```python
from build123d import *

# Parameters (mm, degrees)
BOSS_EXTRUDE1_DEPTH        = 40.48125
SKETCH3_R                  = 6.35
BOSS_EXTRUDE2_DEPTH        = 7.9375
F_10_32_TAPPED_HOLE1_D     = 4.0386
F_10_32_TAPPED_HOLE1_DEPTH = 12.02944
F_10_32_TAPPED_HOLE1_TIP   = 1.213317848
SKETCH2_R                  = 2.0193
CUT_EXTRUDE1_DEPTH         = 90.388013306


with BuildPart() as part:
    # Sketch1 → Boss-Extrude1 (new, symmetric)
    with BuildSketch(Plane(origin=(0, 0, 0), x_dir=(1, 0, 0), z_dir=(0, 1, 0))):
        with BuildLine():
            ThreePointArc((0.990636919, 6.760403927), (0, 6.8326), (-0.990636919, 6.760403927))
            Line((-0.990636919, 6.760403927), (-5.359363081, 4.238118701))
            ThreePointArc((-5.359363081, 4.238118701), (-5.917205174, 3.4163), (-6.35, 2.522285226))
            Line((-6.35, 2.522285226), (-6.35, -2.522285226))
            ThreePointArc((-6.35, -2.522285226), (-5.917205174, -3.4163), (-5.359363081, -4.238118701))
            Line((-5.359363081, -4.238118701), (-0.990636919, -6.760403927))
            ThreePointArc((-0.990636919, -6.760403927), (0, -6.8326), (0.990636919, -6.760403927))
            Line((0.990636919, -6.760403927), (5.359363081, -4.238118701))
            ThreePointArc((5.359363081, -4.238118701), (5.917205174, -3.4163), (6.35, -2.522285226))
            Line((6.35, -2.522285226), (6.35, 2.522285226))
            ThreePointArc((6.35, 2.522285226), (5.917205174, 3.4163), (5.359363081, 4.238118701))
            Line((5.359363081, 4.238118701), (0.990636919, 6.760403927))
        make_face()
    extrude(amount=BOSS_EXTRUDE1_DEPTH, both=True)

    # Sketch3 → Boss-Extrude2 (add)
    with BuildSketch(Plane(origin=(0, 40.48125, 0), x_dir=(1, 0, 0), z_dir=(0, 1, 0))):
        with Locations(Location((0, 0, 0), (0, 0, 60))):
            Circle(SKETCH3_R)
    extrude(amount=BOSS_EXTRUDE2_DEPTH)

    # #10-32 Tapped Hole1
    with Locations(Plane(origin=(0, -40.48125, 0), x_dir=(-1, 0, 0), z_dir=(0, -1, 0))):
        with Locations((0, 0)):
            Hole(F_10_32_TAPPED_HOLE1_D / 2, depth=F_10_32_TAPPED_HOLE1_DEPTH)
            with Locations((0, 0, -(F_10_32_TAPPED_HOLE1_DEPTH + F_10_32_TAPPED_HOLE1_TIP / 2))):  # 118° drill point
                Cone(0, F_10_32_TAPPED_HOLE1_D / 2, F_10_32_TAPPED_HOLE1_TIP, mode=Mode.SUBTRACT)

    # Sketch2 → Cut-Extrude1 (cut, through all)
    with BuildSketch(Plane(origin=(0, -40.48125, 0), x_dir=(1, 0, 0), z_dir=(0, 1, 0))):
        with Locations(Location((0, 0, 0), (0, 0, 90))):
            Circle(SKETCH2_R)
    extrude(amount=CUT_EXTRUDE1_DEPTH, mode=Mode.SUBTRACT)


solid = part.part
```
Could you check a few things on this model? Use its own coordinates, in mm. A direction names the side the tool comes from. Give positions to 0.01 mm unless a question says otherwise; leave off trailing zeros. Loops run counter-clockwise (first coordinate to the right, second up) from the corner with the lowest first, then second, coordinate; pieces in that order, holes last. Notation, with made-up numbers: (42.5, -12.5) -> (94.5, -12.5) arc R37 ccw to (94.5, 24.5) -> close; hole circle Ø2 at (31.25, 73). An arc over 180 degrees is marked (long way). Put each result on its own line as item: value.
(1) Imagine slicing it at C-C on z = -1. Write out the boundary of the cut face in (x, y), plus the area to 3 significant figures.
Computed:
outline: (-6.35, -40.48) -> (-1.75, -40.48) -> (-1.75, 48.42) -> (-6.27, 48.42) -> (-6.27, 40.48) -> (-6.35, 40.48) -> close; (1.75, -40.48) -> (6.35, -40.48) -> (6.35, 40.48) -> (6.27, 40.48) -> (6.27, 48.42) -> (1.75, 48.42) -> close
area: 816 mm^2
(2) Imagine slicing it at A-A on x = 0. Write out the boundary of the cut face in (y, z).
Computed:
outline: (-40.48, -6.83) -> (40.48, -6.83) -> (40.48, -6.35) -> (48.42, -6.35) -> (48.42, -2.02) -> (-40.48, -2.02) -> close; (-40.48, 2.02) -> (48.42, 2.02) -> (48.42, 6.35) -> (40.48, 6.35) -> (40.48, 6.83) -> (-40.48, 6.83) -> close
(3) Imagine slicing it at B-B on y = -16.5. Write out the boundary of the cut face in (x, z), plus the area to 3 significant figures.
Computed:
outline: (-6.35, -2.52) arc R6.83 ccw to (-5.36, -4.24) -> (-0.99, -6.76) arc R6.83 ccw to (0.99, -6.76) -> (5.36, -4.24) arc R6.83 ccw to (6.35, -2.52) -> (6.35, 2.52) arc R6.83 ccw to (5.36, 4.24) -> (0.99, 6.76) arc R6.83 ccw to (-0.99, 6.76) -> (-5.36, 4.24) arc R6.83 ccw to (-6.35, 2.52) -> close; hole circle Ø4.04 at (0, 0)
area: 124 mm^2
(4) I'm going to push flat-ended pins straight in: pin 1 Ø1.5 at (x, y) = (3.5, -8.5) entering from +Z; pin 2 Ø3.5 at (x, z) = (0, 0) entering from +Y; pin 3 Ø1 at (x, y) = (3, 18) entering from -Z. Where does each tip first touch, or does it pass through?
Computed:
pin 1: z = 5.74
pin 2: through
pin 3: z = -5.89
(5) Please list where these lines run through material, in increasing order: probe 1 along X at (y, z) = (22, 0); probe 2 along Z at (x, y) = (0.5, 13.5); probe 3 along X at (y, z) = (-19, -1.25). Write a range as [from, to].
Computed:
probe 1: [-6.35, -2.02], [2.02, 6.35]
probe 2: [-6.81, -1.96], [1.96, 6.81]
probe 3: [-6.35, -1.59], [1.59, 6.35]
(6) For faces 1 (the face through (-5.6, 40.481, 3.3)), 2 (the face through (1.38, 44.39, -6.2)), 3 (the face through (5.7, 40.481, -3.2)), 4 (the face through (5.6, 40.481, 3.3)), which set-ups out of +Z, -Z, +X, -X, +Y, -Y let a thin tool reach every point of the face, with its end or its side?
Computed:
face 1: +Z, -X, +Y
face 2: +Y
face 3: -Z, +X, +Y
face 4: +Z, +X, +Y
(7) Imagine slicing it at D-D on x = -4. Write out the boundary of the cut face in (y, z).
Computed:
outline: (-40.48, -5.02) -> (40.48, -5.02) -> (40.48, -4.93) -> (48.42, -4.93) -> (48.42, 4.93) -> (40.48, 4.93) -> (40.48, 5.02) -> (-40.48, 5.02) -> close
